Could you check a few things on this model? Use its own coordinates, in mm. Face numbers are marked on the shaded views. A direction names the side the tool comes from. Give positions to 0.01 mm unless a question says otherwise; leave off trailing zeros. Loops run counter-clockwise (first coordinate to the right, second up) from the corner with the lowest first, then second, coordinate; pieces in that order, holes last. Notation, with made-up numbers: M -10.5,-24 L 36.5,-24 A26 ccw 36.5,4 Z; hole C -10,40 d10. An arc over 180 degrees is marked long. Return JSON: item names as keys, results as strings. Group by question number.
1. For the marked faces 1, 2 and 3, which set-ups out of +Z, -Z, +X, -X, +Y, -Y let a thin tool reach every point of the face, with its end or its side?
2. If we mould it in two halves opening along Y, with no side actions, what happens to the marked faces 4, 5 and 6? For each: +Y half, -Y half, draft (parallel to the pull), parting line (faces both ways), or undercut.
3. If we section it at C-C (z = 20): Write out the boundary of the cut face in (x, y), plus the area to 3 significant figures.
4. Please list where these lines run through material, in increasing order: line 1 (Y direction, x = 17, z = 27); line 2 (X direction, y = 16, z = 21); line 3 (Y direction, x = 25.5, z = 24).
5. If we section it at A-A (y = 15): Write out the boundary of the cut face in (x, z).
6. If we section it at B-B (x = 19): Write out the boundary of the cut face in (y, z).
7. If we section it at D-D (x = 3.5): Write out the boundary of the cut face in (y, z), plus the area to 3 significant figures.
```python
from build123d import *

# Parameters (mm, degrees)
F1_DEPTH = 30
F3_DEPTH = 28


with BuildPart() as f1:
    # F0 (on Top) → F1 (new body)
    with BuildSketch(Plane.XY):
        Polygon((0, 60), (0, 0), (7, 0), (7, 20), (23, 20), (23, 0), (28, 0), (28, 60), align=None)
    extrude(amount=F1_DEPTH)

    # F2 (on face) → F3 (cut, through all)
    with BuildSketch(Plane(origin=(0, 0, 0), x_dir=(0, -1, 0), z_dir=(-1, 0, 0))):
        with BuildLine():
            ThreePointArc((-50, 15), (-40, 5), (-30, 15))
            Line((-30, 15), (-50, 15))
        make_face()
        with BuildLine():
            Line((-50, 15), (-30, 15))
            ThreePointArc((-30, 15), (-40, 25), (-50, 15))
        make_face()
        with BuildLine():
            Line((-30, 15), (-30, 30))
            Line((-30, 30), (-50, 30))
            Line((-50, 30), (-50, 15))
            ThreePointArc((-50, 15), (-40, 25), (-30, 15))
        make_face()
    extrude(amount=-F3_DEPTH, mode=Mode.SUBTRACT)

    # F2 (on face) → F4 (revolve, cut)
    with BuildSketch(Plane(origin=(0, 0, 0), x_dir=(0, -1, 0), z_dir=(-1, 0, 0))):
        with BuildLine():
            ThreePointArc((-50, 15), (-40, 5), (-30, 15))
            Line((-30, 15), (-50, 15))
        make_face()
        with BuildLine():
            Line((-49.0138781887, 0), (-30.9861218113, 0))
            ThreePointArc((-30.9861218113, 0), (-24.7685708435, 6.3829491211), (-22.5, 15))
            Line((-22.5, 15), (-30, 15))
            ThreePointArc((-30, 15), (-40, 5), (-50, 15))
            Line((-50, 15), (-57.5, 15))
            ThreePointArc((-57.5, 15), (-55.2314291565, 6.3829491211), (-49.0138781887, 0))
        make_face()
        with BuildLine():
            ThreePointArc((-49.0138781887, 0), (-40, -2.5), (-30.9861218113, 0))
            Line((-30.9861218113, 0), (-49.0138781887, 0))
        make_face()
    revolve(axis=Axis((0, 40, 15), (0, -1, 0)), mode=Mode.SUBTRACT)


solid = f1.part
```
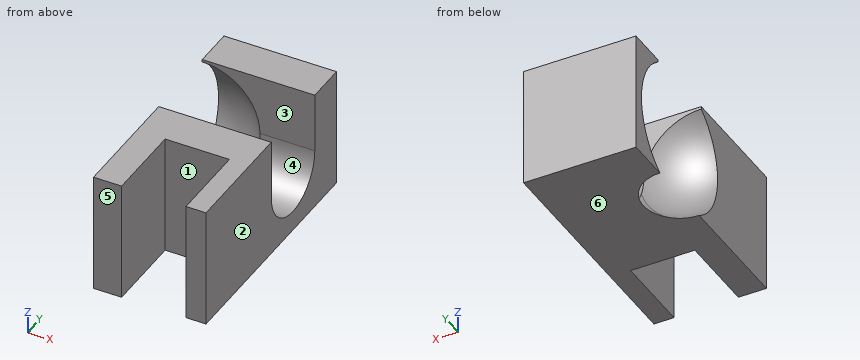
Answer:
{
 "1": {"face 1": "+Z, -Z, -Y", "face 2": "+Z, -Z, +X, +Y, -Y", "face 3": "+Z, +X, -X"},
 "2": {"face 4": "undercut", "face 5": "-Y half", "face 6": "draft"},
 "3": {"outline": "M 0,0 L 7,0 L 7,20 L 23,20 L 23,0 L 28,0 L 28,30 L 13.46,30 A16.77 cw 0,23.23 Z; M 0,56.77 A16.77 cw 13.46,50 L 28,50 L 28,60 L 0,60 Z", "area": "673 mm²"},
 "4": {"line 1": "y = 20 to 30, 50 to 60", "line 2": "x = 0 to 7, 23 to 28", "line 3": "y = 0 to 30, 50 to 60"},
 "5": {"outline": "M 0,0 L 7,0 L 7,30 L 0,30 Z; M 23,0 L 28,0 L 28,30 L 23,30 Z"},
 "6": {"outline": "M 20,0 L 60,0 L 60,30 L 50,30 L 50,15 A10 cw 30,15 L 30,30 L 20,30 Z"},
 "7": {"outline": "M 0,0 L 31.69,0 A17.15 cw 30,28.93 L 30,30 L 0,30 Z; M 48.31,0 L 60,0 L 60,30 L 50,30 L 50,28.93 A17.15 cw Z", "area": "923 mm²"}
}
